Source: three-view drawing plus pictorial views. Frame: mm from the lowest corner of the part. Give positions to 0.01 mm unless a question says otherwise; leave off trailing zeros. Answer in a Markdown table with one row per item. Add a question column.
1. Ray query, line 1 (X direction, y = 5, z = 6.35) (1 decimal); line 2 (Y direction, x = 9.75, z = 19.5); line 3 (X direction, y = 3, z = 6.35) (1 decimal). Return the intervals inside material, ascending. Write a range as [from, to].
2. Section query A-A on y = 4.25. Count the separate pieces of the cut face and the enclosed holes in it, and give its area (3 significant figures).
3. Contact query for flat-ended pins moving along their axis: pin 1 (5 mm diameter, centred on x = 3.5, z = 26.5, fed in from +Y); pin 2 (8 mm diameter, centred on x = 16, z = 23, fed in from -Y); pin 3 (1.6 mm diameter, centred on x = 9, z = 32, fed in from -Y). Output: stop coordinate, or through.
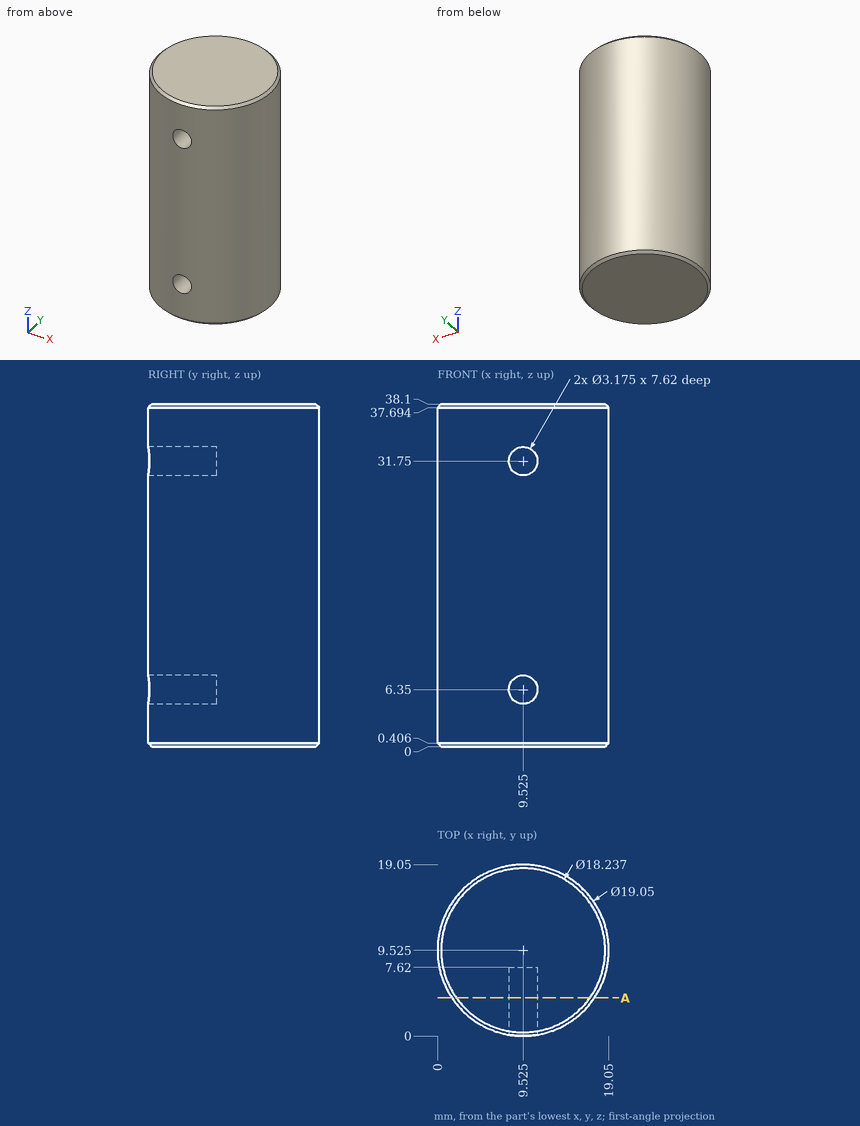
Answer:
| question | item | result |
|---|---|---|
| 1 | line 1 | x = [1.1, 7.9], [11.1, 17.9] |
| 1 | line 2 | y = [0, 19.05] |
| 1 | line 3 | x = [2.6, 7.9], [11.1, 16.5] |
| 2 | separate pieces | 1 |
| 2 | enclosed holes | 2 |
| 2 | area | 588 mm² |
| 3 | pin 1 | stops at y = 18.37 |
| 3 | pin 2 | stops at y = 0.33 |
| 3 | pin 3 | stops at y = 7.62 |
